Geometry: final body of the model. Coordinates: model frame, mm. A direction names the side the tool comes from. Coordinates: 2 decimals unless noted, no trailing zeros. Order: outer loops, then holes, each group sorted by start corner. A loop starts at its lowest first (then second) coordinate and runs counter-clockwise, first axis right, second up. Notation, with made-up numbers: (61.25, 34) -> (69.25, 34) arc R31 ccw to (69.25, 61) -> close; hole circle Ø6 at (-22.75, 15.5). An arc over 180 degrees is marked (long way). Use CSV: the item, a comma, the result in double quotes. Start each with the question number.
Autodesk Fusion 360 part; units mm, degrees
sketch "Sketch1" plane through (0, 0, 0) normal (0, 1, 0) x (1, 0, 0)
  line L0 (2.1997, -3.81) -> (35.9003, -62.1811)
  line L1 (4.3994, 0) -> (71.8006, 0) construction
  line L2 (40.2997, -62.1811) -> (74.0003, -3.81)
  line L3 (76.2, 0) -> (0, 0)
  arc A0 (35.9003, -62.1811) -> (40.2997, -62.1811) centre (38.1, -60.9111) ccw
  arc A1 (74.0003, -3.81) -> (71.8006, 0) centre (71.8006, -2.54) ccw
  arc A2 (4.3994, 0) -> (2.1997, -3.81) centre (4.3994, -2.54) ccw
  point P0 (38.1, -65.9911)
  point P1 (76.2, 0)
  dimension "d1" = 60
  dimension "d2" = 76.2
  dimension "d4" = 76.2
  dimension "d7" = 2.54
  dimension "d8" = 2.54
extrude "Extrude1" add sketch "Sketch1" along normal blind 12.7
sketch "Sketch2" plane through (0, 0, 0) normal (0, -1, 0) x (1, 0, 0)
  arc A0 (2.1997, 3.81) -> (4.3994, 0) centre (4.3994, 2.54) ccw
  line L0 (4.3994, 0) -> (71.8006, 0)
  arc A1 (71.8006, 0) -> (74.0003, 3.81) centre (71.8006, 2.54) ccw
  line L1 (74.0003, 3.81) -> (40.2997, 62.1811)
  arc A2 (40.2997, 62.1811) -> (35.9003, 62.1811) centre (38.1, 60.9111) ccw
  line L2 (35.9003, 62.1811) -> (2.1997, 3.81)
  circle A3 centre (38.1, 12.7) radius 3.175
  line L3 (31.2844, 35.295) -> (26.7797, 35.295)
  arc A4 (43.8189, 35.3736) -> (31.8923, 35.7466) centre (37.8056, 33.9623) ccw
  arc A5 (50.3635, 32.7617) -> (26.1659, 36.0926) centre (38.0602, 32.9416) ccw
  arc A6 (39.4129, 29.0927) -> (43.8356, 35.2148) centre (37.1886, 35.3581) ccw
  arc A7 (45.1318, 26.343) -> (50.3389, 32.5958) centre (40.6355, 35.382) ccw
  arc A8 (39.4129, 29.0927) -> (34.8601, 19.4443) centre (44.4732, 20.8065) ccw
  arc A9 (45.1318, 26.343) -> (41.228, 19.5734) centre (48.2777, 20.0185) ccw
  line L4 (35.4888, 18.8984) -> (40.5943, 18.8984)
  arc A10 (26.1659, 36.0926) -> (26.7797, 35.295) centre (26.7797, 35.93) ccw
  arc A11 (31.2844, 35.295) -> (31.8923, 35.7466) centre (31.2844, 35.93) ccw
  arc A12 (34.8601, 19.4443) -> (35.4888, 18.8984) centre (35.4888, 19.5334) ccw
  arc A13 (40.5943, 18.8984) -> (41.228, 19.5734) centre (40.5943, 19.5334) ccw
  arc A14 (43.8356, 35.2148) -> (43.8189, 35.3736) centre (43.2007, 35.2285) ccw
  arc A15 (50.3389, 32.5958) -> (50.3635, 32.7617) centre (49.7286, 32.771) ccw
  point P0 (34.9534, 18.8984)
  point P1 (41.3034, 18.8984)
  dimension "d9" = 6.35
  dimension "d11" = 6.35
  dimension "d12" = 0.635
extrude "Extrude2" cut 1 faces at (38.8332, 12.7, 20.727) along direction (0, -1, 0) blind 2.54
extrude "Extrude3" cut sketch "Sketch2" against normal blind 2.54 contours A3 | L3 A4 A5 A6 A7 A8 A9 L4 A10 A11 A12 A13 A14 A15
fillet "Fillet1" radius 1.27 6 edges at (38.1, 0, 0) (2.1997, 0, 1.27) (19.05, 0, 32.9956) (38.1, 0, 63.4511) (57.15, 0, 32.9956) (74.0003, 0, 1.27)
fillet "Fillet2" radius 1.27 6 edges at (19.05, 10.16, 32.9956) (2.1997, 10.16, 1.27) (38.1, 10.16, 0) (74.0003, 10.16, 1.27) (57.15, 10.16, 32.9956) (38.1, 10.16, 63.4511)
(1) First-contact query: pin 1 (3 mm diameter, centred on y = 2, z = 21.5, fed in from -X); pin 2 (0.8 mm diameter, centred on x = 30, y = 0.5, fed in from +Z); pin 3 (2 mm diameter, centred on y = 6, z = 47.5, fed in from +X). Flat tips, straight axial feed; report the tip coordinate or a pass-through.
(2) Mould query, pull axis Z, two halves, no side actions, for faces 3 (the face through (39, 5, 0)), 4 (the face through (57.07, 0.38, 32.41)), 5 (the face through (2.181, 5.027, 1.302)), 6 (the face through (38, 1, 18.898)). Classes: pulls with the +Z half, pulls with the -Z half, needs draft (parallel to the pull), parting line crosses it, or undercut.
(3) Line query: line 1 (Z direction, x = 38.1, y = 1.1) (3 decimals); line 2 (Z direction, x = 38.1, y = 0.8) (3 decimals); line 3 (Z direction, x = 61, y = 7). Output: solid intervals per line, ascending. Write a range as from..to.
(4) Access query for faces 1 (the face through (19.62, 9.8, 33.21)), 2 (the face through (35.727, 1.252, 25.021)). Directions: +Z, -Z, +X, -X, +Y, -Y. A direction counts if a zero-diameter tool reaches every point of the face in a straight line with its end or side. Return the directions, or none.
(5) Section A-A (y = 4.5). Return loops of the section in (x, z), then the cut area to 3 significant figures.
Check sheet entries:
1,pin 1,"stops at x = 11.55"
1,pin 2,"stops at z = 52.29"
1,pin 3,"stops at x = 49.35"
2,face 3,"pulls with the -Z half"
2,face 4,"pulls with the +Z half"
2,face 5,"parting line crosses it"
2,face 6,"undercut"
3,line 1,"z = 0.011..9.525, 15.875..18.898, 28.131..40.132, 45.246..63.44"
3,line 2,"z = 0.09..9.525, 15.875..18.898, 28.131..40.132, 45.246..63.361"
3,line 3,"z = 0..26.33"
4,face 1,"+Z, -X, +Y"
4,face 2,"-Y"
5,outline,"(2.2, 3.81) arc R2.54 ccw to (4.4, 0) -> (71.8, 0) arc R2.54 ccw to (74, 3.81) -> (40.3, 62.18) arc R2.54 ccw to (35.9, 62.18) -> close"
5,area,"2,500 mm^2"
